Read the model definition and answer for the solid it produces. Units are mm, in the model's axes. A direction names the side the tool comes from. Coordinates: 2 decimals unless noted, no trailing zeros. Return JSON: item names as keys, results as strings.
from build123d import *

# Parameters (mm, degrees)
P_IDAT_VYSUNUT_M3_DEPTH  = 2
SKICA5_W                 = 19
SKICA5_H                 = 32.5
P_IDAT_VYSUNUT_M4_DEPTH  = 1.5
SKICA6_W                 = 1.5
SKICA6_H                 = 13
P_IDAT_VYSUNUT_M5_DEPTH  = 17.75
SKICA6_4_W               = 1.2
SKICA6_4_H               = 9
P_IDAT_VYSUNUT_M6_DEPTH  = 16.75
SKICA9_W                 = 1.3
SKICA9_H                 = 1.369535349
SKICA9_H_2               = 1.34
P_IDAT_VYSUNUT_M7_DEPTH  = 3.2
ODEBRAT_VYSUNUT_M5_DEPTH = 1.2
ODEBRAT_VYSUNUT_M6_DEPTH = 1.5
SKICA13_W                = 7
SKICA13_H                = 14.8
ODEBRAT_VYSUNUT_M7_DEPTH = 2
P_IDAT_VYSUNUT_M9_DEPTH  = 7


with BuildPart() as part:
    # Skica3 → Přidat vysunutím3 (new body)
    with BuildSketch(Plane.XY):
        with BuildLine():
            Line((0, 0), (25, 8.027622297))
            add(Edge.make_bspline(
                [(25, 8.027622297), (25.362983363, 40.405597735), (30, 72.39878495)],
                knots=[0, 0, 0, 1, 1, 1], degree=2))
            add(Edge.make_bspline(
                [(30, 72.39878495), (25.810182082, 106.393156288), (0, 108.597151184)],
                knots=[0, 0, 0, 1, 1, 1], degree=2))
            add(Edge.make_bspline(
                [(-30, 72.39878495), (-25.810182082, 106.393156288), (0, 108.597151184)],
                knots=[0, 0, 0, 1, 1, 1], degree=2))
            add(Edge.make_bspline(
                [(-25, 8.027622297), (-25.362983363, 40.405597735), (-30, 72.39878495)],
                knots=[0, 0, 0, 1, 1, 1], degree=2))
            Line((-25, 8.027622297), (0, 0))
        make_face()
    extrude(amount=P_IDAT_VYSUNUT_M3_DEPTH)

    # Skica5 → Přidat vysunutím4 (add)
    with BuildSketch(Plane.XY.offset(2)):
        with Locations((0, 66.25)):
            Rectangle(SKICA5_W, SKICA5_H)
        Polygon((-8.5, 81.5), (8.5, 81.5), (8.5, 51), (0, 51), (-8.5, 51), align=None, mode=Mode.SUBTRACT)
    extrude(amount=P_IDAT_VYSUNUT_M4_DEPTH)

    # Skica6 → Přidat vysunutím5 (add)
    with BuildSketch(Plane.XY.offset(2)):
        with Locations((-6.95, 28.5)):
            Rectangle(SKICA6_W, SKICA6_H)
    extrude(amount=P_IDAT_VYSUNUT_M5_DEPTH)

    # Skica6<4> → Přidat vysunutím6 (add)
    with BuildSketch(Plane.XY.offset(2)):
        with Locations((7.4, 29.16)):
            Rectangle(SKICA6_4_W, SKICA6_4_H)
    extrude(amount=P_IDAT_VYSUNUT_M6_DEPTH)

    # Skica9 → Přidat vysunutím7 (add)
    with BuildSketch(Plane.XY.offset(2)):
        Polygon((8, 33.659998668), (8, 32.477114588), (9.4, 32.477114544), (9.4, 33.659998668), align=None)
        Polygon((8, 24.659998668), (8, 25.841591632), (9.399999793, 25.841591589), (9.399999793, 24.659998668), align=None)
        with Locations((-8.35, 22.684767675)):
            Rectangle(SKICA9_W, SKICA9_H)
        with Locations((-8.35, 34.33)):
            Rectangle(SKICA9_W, SKICA9_H_2)
    extrude(amount=P_IDAT_VYSUNUT_M7_DEPTH)

    # Skica11 → Odebrat vysunutím5 (cut)
    with BuildSketch(Plane(origin=(8, 0, 0), x_dir=(0, 0, -1), z_dir=(1, 0, 0))):
        with BuildLine():
            Line((-18.75, 27.56), (-18.75, 30.76))
            Line((-18.75, 30.76), (-14.8, 30.76))
            ThreePointArc((-14.8, 30.76), (-13.2, 29.16), (-14.8, 27.56))
            Line((-14.8, 27.56), (-18.75, 27.56))
        make_face()
    extrude(amount=-ODEBRAT_VYSUNUT_M5_DEPTH, mode=Mode.SUBTRACT)

    # Skica12 → Odebrat vysunutím6 (cut)
    with BuildSketch(Plane.ZY.offset(7.7)):
        with BuildLine():
            Line((19.75, 32.1), (19.75, 24.9))
            Line((19.75, 24.9), (15.6, 24.9))
            ThreePointArc((15.6, 24.9), (12, 28.5), (15.6, 32.1))
            Line((15.6, 32.1), (19.75, 32.1))
        make_face()
    extrude(amount=-ODEBRAT_VYSUNUT_M6_DEPTH, mode=Mode.SUBTRACT)

    # Skica13 → Odebrat vysunutím7 (cut)
    with BuildSketch(Plane.XY.offset(2)):
        with Locations((0, 70.9)):
            Rectangle(SKICA13_W, SKICA13_H)
    extrude(amount=-ODEBRAT_VYSUNUT_M7_DEPTH, mode=Mode.SUBTRACT)

    # Skica15 → Přidat vysunutím9 (add)
    with BuildSketch(Plane.XY.offset(2)):
        with BuildLine():
            Line((-23.017222129, 9.491521925), (0, 2.100579303))
            Line((0, 2.100579303), (23.017222129, 9.491521925))
            add(Edge.make_bspline(
                [(23.017222129, 9.491521925), (23.104228084, 14.820015615), (23.412919749, 25.481851116), (24.427384602, 41.413676681), (25.947336757, 57.30526528), (27.328834525, 67.881140695), (28.08811969, 73.155746738)],
                knots=[-0.017295959, -0.017295959, -0.017295959, -0.017295959, 0.240841414, 0.498978787, 0.75711616, 1.015253532, 1.015253532, 1.015253532, 1.015253532], degree=3))
            Line((28.08811969, 73.155746738), (26.468325097, 72.43096677))
            add(Edge.make_bspline(
                [(21.534974927, 10.590999575), (21.873259628, 31.308522725), (23.516034404, 51.921978771), (26.468325097, 72.43096677)],
                knots=[0, 0, 0, 0, 1, 1, 1, 1], degree=3))
            Line((21.534974927, 10.590999575), (0, 3.676013779))
            Line((0, 3.676013779), (-21.534974927, 10.590999575))
            add(Edge.make_bspline(
                [(-26.468325097, 72.43096677), (-23.516034403, 51.921978771), (-21.873259627, 31.308522725), (-21.534974927, 10.590999575)],
                knots=[0, 0, 0, 0, 1, 1, 1, 1], degree=3))
            Line((-26.468325097, 72.43096677), (-28.08811969, 73.15574674))
            add(Edge.make_bspline(
                [(-28.08811969, 73.15574674), (-27.328834525, 67.881140697), (-25.947336757, 57.305265281), (-24.427384601, 41.413676681), (-23.412919749, 25.481851116), (-23.104228084, 14.820015615), (-23.017222129, 9.491521925)],
                knots=[-0.015253532, -0.015253532, -0.015253532, -0.015253532, 0.24288384, 0.501021213, 0.759158586, 1.017295959, 1.017295959, 1.017295959, 1.017295959], degree=3))
        make_face()
    extrude(amount=P_IDAT_VYSUNUT_M9_DEPTH)


solid = part.part
1. The part is cut by section A-A (z = 7.5). Count the separate pieces of the cut face and the enclosed holes in it, then the cut area to 3 significant figures.
Taken from the geometry:
{"separate pieces": "3", "enclosed holes": "0", "area": "290 mm2"}
2. A tool of negligible diameter and unlimited length cuts with its end or side. For faces 5 (the face through (3.5, 71, 1)), 6 (the face through (-10.617, 7.085, 5.451)), 7 (the face through (-9, 66, 3.5)), 8 (the face through (-11.67, 5.848, 5.451)), from which of +Z, -Z, +X, -X, +Y, -Y can it reach the whole face along a straight path? Write none if from no direction.
Taken from the geometry:
{"face 5": "+Z, -Z", "face 6": "+Z", "face 7": "+Z, +Y", "face 8": "+Z, -X, -Y"}
3. For a pull along X with two mould halves and no side action, classify faces 1 (the face through (-7, 35, 9)), 2 (the face through (11.347, 5.744, 5.451)), 3 (the face through (10.918, 7.182, 5.451)), 4 (the face through (-23, 30, 9)) as +X half, -X half, draft (parallel to the pull), parting line (faces both ways), or undercut.
Taken from the geometry:
{"face 1": "undercut", "face 2": "+X half", "face 3": "undercut", "face 4": "draft"}
4. Flat-ended cylindrical pins translate along their axes: pin 1 Ø1 at (x, y) = (7.5, 26) entering from +Z; pin 2 Ø6 at (x, z) = (-11.5, 13.5) entering from -Y; pin 3 Ø1.3 at (x, z) = (7.5, 16.5) entering from +Y; pin 4 Ø10 at (y, z) = (31, 10) entering from -X. Find the tip coordinate at first contact, or state that the pin passes through.
Taken from the geometry:
{"pin 1": "stops at z = 18.75", "pin 2": "passes through", "pin 3": "stops at y = 33.66", "pin 4": "stops at x = -24.1"}
5. Consider L1, parallel to Y at x = -3.5, z = 2.25; L2, parallel to X at y = 29.5, z = 5.75; L3, parallel to Z at x = -4, y = 48.5. Determine where each line is inside the solid, lowest interval first.
Taken from the geometry:
{"L1": "y = 3.22 to 4.8, 50 to 51, 81.5 to 82.5", "L2": "x = -23.71 to -22.21, -7.7 to -6.2, 6.8 to 8, 22.21 to 23.71", "L3": "z = 0 to 2"}
